Can you work these out from the model? Positions are in its coordinate system, mm. A direction names the side the tool comes from. Give positions to 0.01 mm unless a question says otherwise; leave off trailing zeros. Order: outer loops, then holes, each group sorted by start corner. A loop starts at its lowest first (then second) coordinate and runs counter-clockwise, first axis right, second up.
Item 1: If we mould it in two halves opening along Z, with no side actions, what happens to faces 1 (the flat face through (7, 2, 492.125)), 2 (the flat face through (3.175, 14, 108)), 3 (the flat face through (7, 2, 0))? For each: +Z half, -Z half, draft (parallel to the pull), parting line (faces both ways), or undercut.
Item 2: I want a section at B-B, the plane z = 454. Write out the boundary of the cut face in (x, y) (3 decimals).
Item 3: Which directions (+Z, -Z, +X, -X, +Y, -Y) give clear straight access to the entire face, cutting with the end or side of a thin tool? Please do faces 4 (the flat face through (3.175, 14, 451)), 5 (the flat face through (0, 13, 243)).
Item 4: If I drill on line 1 along Z through (x, y) = (12.7, 1.75) (3 decimals); line 2 along X through (y, z) = (1.05, 12.7); line 3 along Y through (x, z) = (13, 279) (3 decimals), over which ranges is the centre line in solid material (lowest first)?
Item 5: I want a section at C-C, the plane z = 47.5. Write out the boundary of the cut face in (x, y) (3 decimals), then the cut area to 3 significant figures.
Item 6: I want a section at A-A, the plane y = 15.75. Count the separate pieces of the cut face and the enclosed holes in it, then the cut area to 3 significant figures.
Item 7: I'm going to push flat-ended pins straight in: pin 1 Ø11 at (y, z) = (17, 229) entering from +X (3 decimals); pin 2 Ø12.5 at (x, z) = (13, 189) entering from +Y (3 decimals). Where does each tip first touch, or does it pass through?
Autodesk Inventor part; units mm, degrees
ref_plane "YZ Plane" through (0, 0, 0) normal (1, 0, 0) x (0, 1, 0)
ref_plane "XZ Plane" through (0, 0, 0) normal (0, 1, 0) x (-1, 0, 0)
ref_plane "XY Plane" through (0, 0, 0) normal (0, 0, 1) x (1, 0, 0)
sketch "Sketch1" plane through (0, 0, 0) normal (0, 0, 1) x (1, 0, 0)
  line L0 (0, 25.4) -> (0, 0)
  line L1 (0, 0) -> (25.4, 0)
  line L2 (3.175, 25.4) -> (3.175, 4.953)
  line L3 (4.953, 3.175) -> (25.4, 3.175)
  line L4 (0, 25.4) -> (3.175, 25.4)
  line L5 (25.4, 3.175) -> (25.4, 0)
  line L6 (3.175, 4.953) -> (3.175, 3.175)
  line L7 (4.953, 3.175) -> (3.175, 3.175)
  dimension "d0" = 25.4
  dimension "d1" = 25.4
  dimension "d2" = 3.175
extrude "Extrusion1" add sketch "Sketch1" along normal blind 492.125
sketch "Sketch2" plane through (3.175, 3.175, 0) normal (0, 1, 0) x (1, 0, 0)
  circle A0 centre (9.525, -479.425) radius 2.8398
  line L0 (22.225, -492.125) -> (0, -492.125)
  line L1 (22.225, 0) -> (22.225, -492.125)
  circle A1 centre (9.525, -12.7) radius 2.8398
  line L2 (22.225, 0) -> (0, 0)
  point P0 (-3.175, 0)
  point P1 (1.778, -492.125)
  point P2 (1.778, 0)
  dimension "d5" = 12.7
  dimension "d6" = 12.7
  dimension "d9" = 466.725
  dimension "d31" = 12.7
hole "Hole1" at (12.7, 3.175, 479.425) at (12.7, 3.175, 12.7) direction (0, -1, 0) diameter 6.7564 depth 25.4 tip angle 118
sketch "Sketch22" plane through (3.175, 3.175, 0) normal (1, 0, 0) x (0, 0, -1)
  line L0 (0, 22.225) -> (-492.125, 22.225)
  line L1 (0, 0) -> (-492.125, 0)
  line L2 (-414.3375, 22.225) -> (-361.95, 22.225)
  line L3 (-361.95, 22.225) -> (-361.95, 3.175)
  line L4 (-365.125, 0) -> (-411.1625, 0)
  line L5 (-414.3375, 3.175) -> (-414.3375, 22.225)
  line L6 (-492.125, 0) -> (-492.125, 22.225)
  arc A0 (-414.3375, 3.175) -> (-411.1625, 0) centre (-411.1625, 3.175) ccw
  arc A1 (-365.125, 0) -> (-361.95, 3.175) centre (-365.125, 3.175) ccw
  point P0 (0, -3.175)
  point P1 (-361.95, 0)
  point P2 (-414.3375, 0)
  dimension "d137" = 52.3875
  dimension "d138" = 77.7875
  dimension "d139" = 3.175
extrude "Extrusion11" cut sketch "Sketch22" against normal blind 25.4 contours L3 A1 L1 A0 L5 L0
pattern_linear "Rectangular Pattern1" count 4 spacing 111.76 along (0, 0, -1) of "Extrusion11"
Results list:
1. face 1: +Z half
1. face 2: draft
1. face 3: -Z half
2. outline: (0, 0) - (25.4, 0) - (25.4, 3.175) - (3.175, 3.175) - (3.175, 25.4) - (0, 25.4) - close
3. face 4: +Z, -Z, +X, +Y
3. face 5: +Z, -Z, -X, +Y, -Y
4. line 1: z = 0 to 9.322, 16.078 to 476.047, 482.803 to 492.125
4. line 2: x = 0 to 9.32, 16.08 to 25.4
4. line 3: y = 0 to 3.175
5. outline: (0, 0) - (25.4, 0) - (25.4, 3.175) - (0, 3.175) - close
5. area: 80.6 mm2
6. separate pieces: 5
6. enclosed holes: 0
6. area: 897 mm2
7. pin 1: stops at x = 3.175
7. pin 2: stops at y = 3.175
